Geometry check sheet. Reference: drawing and pictorial views, mm from the part's lowest x, y, z. Coordinates: 2 decimals unless noted, no trailing zeros. Loops run counter-clockwise (first coordinate to the right, second up) from the corner with the lowest first, then second, coordinate; pieces in that order, holes last. Notation, with made-up numbers: (76.5, 63) - (107.5, 63) arc R3 ccw to (107.5, 67) - close; hole circle Ø10 at (31, 6.5). An arc over 180 degrees is marked (long way). Use a Markdown table: item, result. Add a question column.
1) Go/stop test with flat-tipped pins: P1, Ø4.5, axis at x = 47.06, z = 15.94, coming from the +Y side; P2, Ø8, axis at x = 16, y = 5.5, coming from the +Z side (1 decimal); P3, Ø1.5, axis at y = 11, z = 34, coming from the +X side; P4, Ø3, axis at x = 42.11, z = 20.89, coming from the +Y side. Record where each tip stops, or that it passes through.
2) Draft check along Z on the marked faces 1, 2 and 3. Enter one of: pulls with the +Z half, pulls with the -Z half, needs draft (parallel to the pull), parting line crosses it, or undercut.
3) Sectioned sample at A-A, the plane y = 9. Enter the section's corners in (x, z), then the cut area to 3 significant figures.
4) Thickness scan on line 1 (Z direction, x = 31.5, y = 0.45); line 2 (Y direction, x = 41, z = 16); line 3 (X direction, y = 11.5, z = 18) (1 decimal). Record the ranges inside material, lowest first.
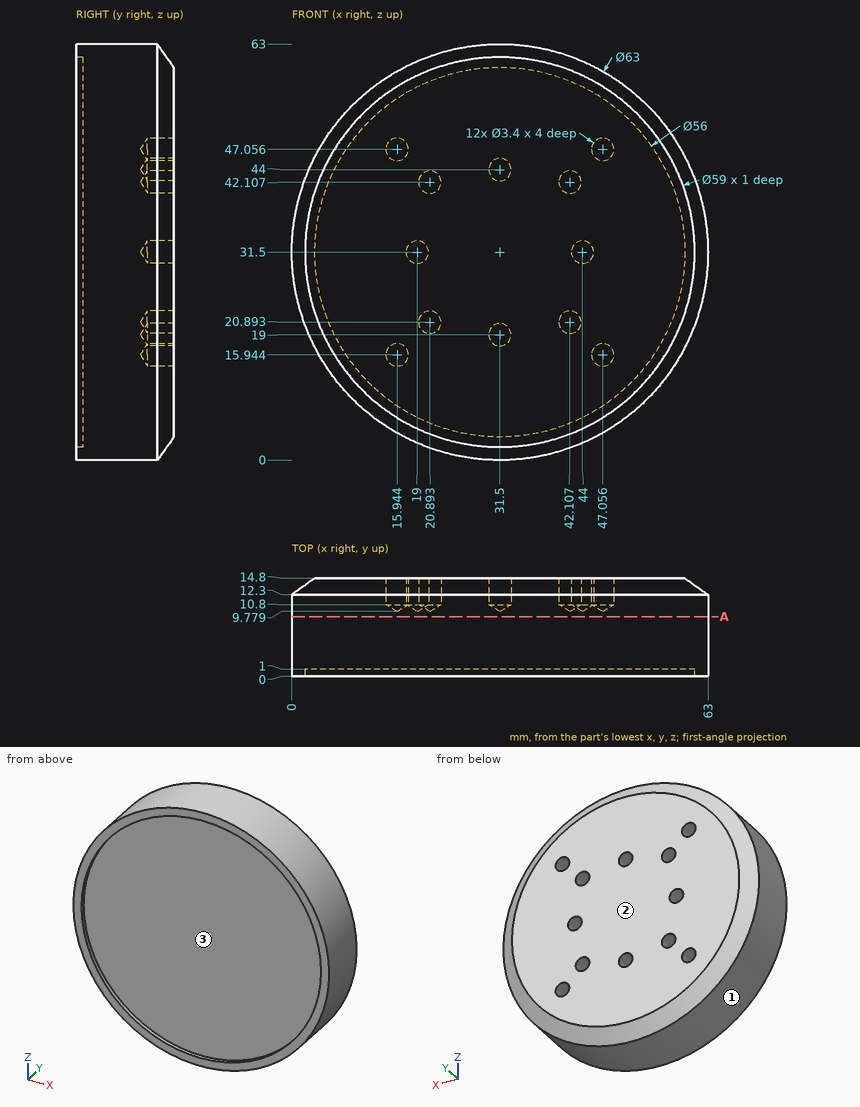
Solved:
| question | item | result |
|---|---|---|
| 1 | P1 | stops at y = 14.8 |
| 1 | P2 | stops at z = 60.8 |
| 1 | P3 | stops at x = 62.95 |
| 1 | P4 | stops at y = 10.68 |
| 2 | face 1 | parting line crosses it |
| 2 | face 2 | needs draft |
| 2 | face 3 | undercut |
| 3 | outline | circle Ø63 at (31.5, 31.5) |
| 3 | area | 3,120 mm2 |
| 4 | line 1 | z = 0 to 2, 61 to 63 |
| 4 | line 2 | y = 1 to 14.8 |
| 4 | line 3 | x = 3 to 30.1, 32.9 to 60 |
